Geometry check sheet. Reference: the model listing, model coordinates, mm. A direction names the side the tool comes from. Round coordinates to 2 decimals unless told otherwise and drop trailing zeros. Write each loop counter-clockwise with the first axis right and the second up, starting at its lowest first coordinate (ties: lowest second). Pieces come first, ordered by that corner, then holes. Notation, with made-up numbers: (42.25, 16.25) -> (97.25, 16.25) arc R16 cw to (97.25, 42.25) -> close; hole circle Ø4 at (-26.5, 71). An arc over 180 degrees is marked (long way). Return JSON: item names as keys, results as strings. Group by question number.
from build123d import *

# Parameters (mm, degrees)
SKETCH1_R               = 4.9609375
BOSS_EXTRUDE1_DEPTH     = 101.6
SKETCH2_R               = 3.175
CUT_EXTRUDE1_DEPTH      = 11.16
CUT_EXTRUDE1_DEPTH_BACK = 11.914472708


with BuildPart() as part:
    # Sketch1 → Boss-Extrude1 (new body, symmetric)
    with BuildSketch(Plane(origin=(0, 0, 0), x_dir=(1, 0, 0), z_dir=(0, 1, 0))):
        with BuildLine():
            ThreePointArc((-54.898232946, 10.914472708), (-55.979756859, 9.486084273), (-57.024125462, 8.030308975))
            ThreePointArc((-57.024125462, 8.030308975), (-55.271492218, -9.123122127), (-40.64, 0))
            Line((-40.64, 0), (40.64, 0))
            ThreePointArc((40.64, 0), (55.271492218, -9.123122127), (57.024125462, 8.030308975))
            ThreePointArc((57.024125462, 8.030308975), (55.979756859, 9.486084273), (54.898232946, 10.914472708))
            Line((54.898232946, 10.914472708), (-54.898232946, 10.914472708))
        make_face()
        with Locations((-50.8, 0)):
            Circle(SKETCH1_R, mode=Mode.SUBTRACT)
        with Locations((50.8, 0)):
            Circle(SKETCH1_R, mode=Mode.SUBTRACT)
    extrude(amount=BOSS_EXTRUDE1_DEPTH, both=True)

    # Sketch2 → Cut-Extrude1 (cut, two sides)
    with BuildSketch(Plane.XY) as cut_extrude1_sk:
        with Locations((-23.278917925, 45.299515962)):
            Circle(SKETCH2_R)
        with Locations((23.278917925, 45.299515962)):
            Circle(SKETCH2_R)
        with Locations((23.278917925, -45.299515962)):
            Circle(SKETCH2_R)
        with Locations((-23.278917925, -45.299515962)):
            Circle(SKETCH2_R)
    extrude(amount=CUT_EXTRUDE1_DEPTH, mode=Mode.SUBTRACT)
    extrude(cut_extrude1_sk.sketch, amount=-CUT_EXTRUDE1_DEPTH_BACK, mode=Mode.SUBTRACT)


solid = part.part
1) Mould release check, pull along X, two halves, no side actions. Record for faces 1 (the face through (1, 1, -10.914)), 2 (the face through (45.844, -1.422, -0.218)), 3 (the face through (-55.53, 1.42, 8.99)): +X half, -X half, draft (parallel to the pull), parting line (faces both ways), or undercut.
2) Go/stop test with flat-tipped pins: P1, Ø1.5, axis at y = 12.5, z = -2.5, coming from the +X side; P2, Ø1.5, axis at y = -71, z = -2, coming from the -X side; P3, Ø1.5, axis at x = 31, y = -3, coming from the +Z side; P4, Ø5, axis at x = 23.28, y = 45.3, coming from the -Z side. Record where each tip stops, or that it passes through.
3) Sectioned sample at A-A on x = -50.8. Enter the section's corners in (y, z), and give its area (3 significant figures).
4) Material ranges on probe 1 along X at (y, z) = (-22, -1.5); probe 2 along X at (y, z) = (-7, -1); probe 3 along Z at (x, y) = (-39, 70.5), recorded low to high. Write a range as [from, to].
5) Sectioned sample at C-C on y = 21. Enter the section's corners in (x, z).
6) Sectioned sample at B-B on z = -3. Enter the section's corners in (x, y) (3 decimals).
7) Tool access check on faces 4 (the face through (24.74, 42.48, -5.38)), 5 (the face through (-1, 1, 0)). Record the directions out of +Z, -Z, +X, -X, +Y, -Y that give a thin tool (end or side, any length) a straight path to the whole face; none if there is none.
8) Sectioned sample at D-D on z = 8. Enter the section's corners in (x, y), and give its area (3 significant figures).
Evaluation:
{
 "1": {"face 1": "draft", "face 2": "undercut", "face 3": "undercut"},
 "2": {"P1": "stops at x = 60.81", "P2": "stops at x = -60.88", "P3": "stops at z = 0", "P4": "passes through"},
 "3": {"outline": "(-101.6, -10.91) -> (101.6, -10.91) -> (101.6, -4.96) -> (-101.6, -4.96) -> close; (-101.6, 4.96) -> (101.6, 4.96) -> (101.6, 10.16) -> (-101.6, 10.16) -> close", "area": "2,270 mm2"},
 "4": {"probe 1": "x = [-60.85, -55.53], [-46.07, 46.07], [55.53, 60.85]", "probe 2": "x = [-60.91, -55.66], [-45.94, 45.94], [55.66, 60.91]", "probe 3": "z = [-10.91, 0]"},
 "5": {"outline": "(-57.02, -8.03) arc R69.54 ccw to (-54.9, -10.91) -> (54.9, -10.91) arc R69.54 ccw to (57.02, -8.03) arc R10.16 ccw (long way) to (40.64, 0) -> (-40.64, 0) arc R10.16 ccw (long way) to start; hole circle Ø9.92 at (-50.8, 0); hole circle Ø9.92 at (50.8, 0)"},
 "6": {"outline": "(-60.507, -101.6) -> (-54.751, -101.6) -> (-54.751, 101.6) -> (-60.507, 101.6) -> close; (-46.849, -101.6) -> (46.849, -101.6) -> (46.849, 101.6) -> (-46.849, 101.6) -> close; (54.751, -101.6) -> (60.507, -101.6) -> (60.507, 101.6) -> (54.751, 101.6) -> close; hole circle Ø6.35 at (-23.279, -45.3); hole circle Ø6.35 at (-23.279, 45.3); hole circle Ø6.35 at (23.279, -45.3); hole circle Ø6.35 at (23.279, 45.3)"},
 "7": {"face 4": "+Z, -Z", "face 5": "+Z, +Y, -Y"},
 "8": {"outline": "(-57.06, -101.6) -> (-44.54, -101.6) -> (-44.54, 101.6) -> (-57.06, 101.6) -> close; (44.54, -101.6) -> (57.06, -101.6) -> (57.06, 101.6) -> (44.54, 101.6) -> close", "area": "5,090 mm2"}
}
